Model file for the job. Use its own axes, mm. A direction names the side the tool comes from. Coordinates: 2 decimals unless noted, no trailing zeros. Order: outer loops, then holes, each group sorted by start corner. A loop starts at its lowest first (then second) coordinate and runs counter-clockwise, first axis right, second up. Notation, with made-up numbers: (41, 38) -> (81, 38) arc R23 ccw to (81, 65) -> close; hole circle Ø10 at (23.25, 84.25). An arc over 180 degrees is marked (long way). Return JSON: item names as keys, results as strings. Group by question number.
1) Which spindle directions (+Z, -Z, +X, -X, +Y, -Y) get a long thin tool onto all of the face, cutting with end or side? Do faces 1 (the cylindrical face through (-72.49, 46.64, 3)), 2 (the flat face through (0, 94.6, 0)). Say none if no direction does.
2) Cut at D-D (x = 60). Write the cut outline in (y, z).
3) Pull direction X, two halves, no side cores. Call faces 3 (the cylindrical face through (84.705, 46.638, -3.83)), 4 (the flat face through (-3, -13, -100)), 5 (the flat face through (200, -13, -1)): +X half, -X half, draft (parallel to the pull), parting line (faces both ways), or undercut.
4) Cut at B-B (x = 0). Write the cut outline in (y, z), and give its area (3 significant figures).
5) Cut at A-A (z = 0). Write the cut outline in (x, y), and give its area (3 significant figures).
6) Cut at C-C (y = 85). Write the cut outline in (x, z).
7) Probe line 1 (X direction, y = 74.5, z = 5.5); line 2 (Y direction, x = 62, z = -14.5); line 3 (Z direction, x = 81, y = 70). List the from-to ranges inside material, lowest first.
8) Flat gauge pins, fed straight in: pin 1 (5 mm diameter, centred on x = 6, y = 21, fed in from +Z); pin 2 (8 mm diameter, centred on x = 29, z = 55, fed in from +Y). Where does each tip first touch, or does it go through?
from build123d import *

# Parameters (mm, degrees)
F0_W     = 400
F0_H     = 200
F1_DEPTH = 25.4
F3_R     = 12.7
F4_R     = 12.7
F2_R     = 10
F5_DEPTH = 120


with BuildPart() as f1:
    # F0 (on Front) → F1 (new body)
    with BuildSketch(Plane.XZ):
        Rectangle(F0_W, F0_H)
    extrude(amount=F1_DEPTH)

    # F3
    f3_edges = [f1.edges().sort_by_distance(p)[0] for p in [
        (-200, -12.7, -100),
        (200, -12.7, -100),
        (200, -12.7, 100),
    ]]
    fillet(f3_edges, radius=F3_R)

    # F4
    f4_edges = [f1.edges().sort_by_distance(p)[0] for p in [
        (-200, -12.7, 100),
    ]]
    fillet(f4_edges, radius=F4_R)

    # F2 (on face) → F5 (join)
    with BuildSketch(Plane.XZ.offset(25.4)):
        with Locations((-82.030319, 0)):
            Circle(F2_R)
        Circle(F2_R)
        with Locations((75.467892, 0)):
            Circle(F2_R)
    extrude(amount=-F5_DEPTH)


solid = f1.part
Answers below:
{
 "1": {"face 1": "+Y", "face 2": "+Z, -Z, +X, -X, +Y"},
 "2": {"outline": "(-25.4, -100) -> (0, -100) -> (0, 100) -> (-25.4, 100) -> close"},
 "3": {"face 3": "undercut", "face 4": "draft", "face 5": "+X half"},
 "4": {"outline": "(-25.4, -100) -> (0, -100) -> (0, -10) -> (94.6, -10) -> (94.6, 10) -> (0, 10) -> (0, 100) -> (-25.4, 100) -> close", "area": "6,970 mm^2"},
 "5": {"outline": "(-200, -25.4) -> (200, -25.4) -> (200, 0) -> (85.47, 0) -> (85.47, 94.6) -> (65.47, 94.6) -> (65.47, 0) -> (10, 0) -> (10, 94.6) -> (-10, 94.6) -> (-10, 0) -> (-72.03, 0) -> (-72.03, 94.6) -> (-92.03, 94.6) -> (-92.03, 0) -> (-200, 0) -> close", "area": "15,800 mm^2"},
 "6": {"outline": "circle Ø20 at (-82.03, 0); circle Ø20 at (0, 0); circle Ø20 at (75.47, 0)"},
 "7": {"line 1": "x = -90.38 to -73.68, -8.35 to 8.35, 67.12 to 83.82", "line 2": "y = -25.4 to 0", "line 3": "z = -8.33 to 8.33"},
 "8": {"pin 1": "stops at z = 9.37", "pin 2": "stops at y = 0"}
}
